from build123d import *

# Parameters (mm, degrees)
F1_DEPTH  = 6
F3_DEPTH  = 0.5
F5_DEPTH  = 0.5
F6_R      = 2.99999
F7_R      = 2.99999
F9_DEPTH  = 2
F10_DEPTH = 0.25
F11_R     = 0.75
F12_DEPTH = 2
F13_DEPTH = 0.25


# Not quite as in the source:
# - a fillet or chamfer is up to 0.001 mm smaller than in the source, because OpenCascade refuses the exact size


with BuildPart() as f1:
    # F0 (on Top) → F1 (new body)
    with BuildSketch(Plane.XY):
        with BuildLine():
            ThreePointArc((-21.257927263, 3.0925971456), (-19.5135237331, 1.2849088277), (-19.5663380414, -1.2266427602))
            ThreePointArc((-19.5663380414, -1.2266427602), (-17.0596555887, 1.5276447909), (-13.757927263, 3.2504758611))
            Line((-13.757927263, 3.2504758611), (-13.757927263, 16.4425971456))
            Line((-13.757927263, 16.4425971456), (-21.257927263, 12.0925971456))
            Line((-21.257927263, 12.0925971456), (-21.257927263, 3.0925971456))
        make_face()
        with BuildLine():
            ThreePointArc((-19.937029438, -1.8621137259), (-13.1593751133, -17.2347921219), (0.092072737, -6.9074028544))
            ThreePointArc((0.092072737, -6.9074028544), (-0.2305379955, -4.3059550041), (-1.178825088, -1.8621137259))
            ThreePointArc((-1.178825088, -1.8621137259), (-1.3821012217, -1.5548376637), (-1.5495164847, -1.2266427602))
            ThreePointArc((-1.5495164847, -1.2266427602), (-4.0561989374, 1.5276447909), (-7.357927263, 3.2504758611))
            Line((-7.357927263, 3.2504758611), (-7.357927263, 1.1925971456))
            Line((-7.357927263, 1.1925971456), (-7.357927263, 0.9928541258))
            Line((-7.357927263, 0.9928541258), (-10.557927263, 0.9928541258))
            Line((-10.557927263, 0.9928541258), (-13.757927263, 0.9928541258))
            Line((-13.757927263, 0.9928541258), (-13.757927263, 1.1925971456))
            Line((-13.757927263, 1.1925971456), (-13.757927263, 3.2504758611))
            ThreePointArc((-13.757927263, 3.2504758611), (-17.0596555887, 1.5276447909), (-19.5663380414, -1.2266427602))
            ThreePointArc((-19.5663380414, -1.2266427602), (-19.7337533043, -1.5548376637), (-19.937029438, -1.8621137259))
        make_face()
        with BuildLine():
            ThreePointArc((-7.407927263, -6.9074028544), (-12.7853136237, -9.1347892152), (-10.557927263, -3.7574028544))
            ThreePointArc((-10.557927263, -3.7574028544), (-8.3305409023, -4.6800164937), (-7.407927263, -6.9074028544))
        make_face(mode=Mode.SUBTRACT)
        with BuildLine():
            ThreePointArc((-7.357927263, 3.2504758611), (-4.0561989374, 1.5276447909), (-1.5495164847, -1.2266427602))
            ThreePointArc((-1.5495164847, -1.2266427602), (-1.6023307929, 1.2849088277), (0.142072737, 3.0925971456))
            Line((0.142072737, 3.0925971456), (0.142072737, 12.0925971456))
            Line((0.142072737, 12.0925971456), (-7.357927263, 16.4425971456))
            Line((-7.357927263, 16.4425971456), (-7.357927263, 3.2504758611))
        make_face()
    extrude(amount=F1_DEPTH)

    # F2 (on face) → F3 (join)
    with BuildSketch(Plane.YZ.offset(-13.757927263)):
        with BuildLine():
            ThreePointArc((11.9425971456, 0), (14.0639174891, 0.8786796564), (14.9425971456, 3))
            ThreePointArc((14.9425971456, 3), (14.0639174891, 5.1213203436), (11.9425971456, 6))
            ThreePointArc((11.9425971456, 6), (8.9425971456, 3), (11.9425971456, 0))
        make_face()
    extrude(amount=F3_DEPTH)

    # F4 (on face) → F5 (join)
    with BuildSketch(Plane(origin=(-7.357927263, 0, 0), x_dir=(0, -1, 0), z_dir=(-1, 0, 0))):
        with BuildLine():
            ThreePointArc((-11.9425971456, 0), (-9.821276802, 0.8786796564), (-8.9425971456, 3))
            ThreePointArc((-8.9425971456, 3), (-9.821276802, 5.1213203436), (-11.9425971456, 6))
            ThreePointArc((-11.9425971456, 6), (-14.9425971456, 3), (-11.9425971456, 0))
        make_face()
    extrude(amount=F5_DEPTH)

    # F6 (radius 3 in the source; OpenCascade refuses exactly that, so slightly less here)
    f6_edges = [f1.edges().sort_by_distance(p)[0] for p in [
        (-10.557927, 0.992854, 0),
        (-10.557927, 0.992854, 6),
    ]]
    fillet(f6_edges, radius=F6_R)

    # F7 (radius 3 in the source; OpenCascade refuses exactly that, so slightly less here)
    f7_edges = [f1.edges().sort_by_distance(p)[0] for p in [
        (-3.607927, 14.267597, 6),
        (-3.607927, 14.267597, 0),
        (-17.507927, 14.267597, 6),
        (-17.507927, 14.267597, 0),
    ]]
    fillet(f7_edges, radius=F7_R)

    # F8 (on face) → F9 (cut)
    with BuildSketch(Plane.XY.offset(6)):
        with BuildLine():
            ThreePointArc((-10.557927263, -13.8074028544), (-12.057927263, -15.3074028544), (-10.557927263, -16.8074028544))
            Line((-10.557927263, -16.8074028544), (-10.557927263, -16.0574028544))
            ThreePointArc((-10.557927263, -16.0574028544), (-11.307927263, -15.3074028544), (-10.557927263, -14.5574028544))
            Line((-10.557927263, -14.5574028544), (-10.557927263, -13.8074028544))
        make_face()
        with BuildLine():
            ThreePointArc((-7.557927263, -13.8074028544), (-8.4366069195, -11.6860825109), (-10.557927263, -10.8074028544))
            ThreePointArc((-10.557927263, -10.8074028544), (-9.057927263, -12.3074028544), (-10.557927263, -13.8074028544))
            Line((-10.557927263, -13.8074028544), (-10.557927263, -14.5574028544))
            ThreePointArc((-10.557927263, -14.5574028544), (-10.0275971771, -14.7770727685), (-9.807927263, -15.3074028544))
            ThreePointArc((-9.807927263, -15.3074028544), (-10.0275971771, -15.8377329403), (-10.557927263, -16.0574028544))
            Line((-10.557927263, -16.0574028544), (-10.557927263, -16.8074028544))
            ThreePointArc((-10.557927263, -16.8074028544), (-8.4366069195, -15.928723198), (-7.557927263, -13.8074028544))
        make_face()
        with BuildLine():
            Line((-10.557927263, -13.0574028544), (-10.557927263, -11.5574028544))
            ThreePointArc((-10.557927263, -11.5574028544), (-11.307927263, -12.3074028544), (-10.557927263, -13.0574028544))
        make_face()
        with BuildLine():
            ThreePointArc((-9.807927263, -12.3074028544), (-10.0275971771, -11.7770727685), (-10.557927263, -11.5574028544))
            Line((-10.557927263, -11.5574028544), (-10.557927263, -13.0574028544))
            ThreePointArc((-10.557927263, -13.0574028544), (-10.0275971771, -12.8377329403), (-9.807927263, -12.3074028544))
        make_face()
    extrude(amount=-F9_DEPTH, mode=Mode.SUBTRACT)

    # F8 (on face) → F10 (cut)
    with BuildSketch(Plane.XY.offset(6)):
        with BuildLine():
            Line((-10.557927263, -11.5574028544), (-10.557927263, -10.8074028544))
            ThreePointArc((-10.557927263, -10.8074028544), (-13.557927263, -13.8074028544), (-10.557927263, -16.8074028544))
            ThreePointArc((-10.557927263, -16.8074028544), (-12.057927263, -15.3074028544), (-10.557927263, -13.8074028544))
            Line((-10.557927263, -13.8074028544), (-10.557927263, -13.0574028544))
            ThreePointArc((-10.557927263, -13.0574028544), (-11.307927263, -12.3074028544), (-10.557927263, -11.5574028544))
        make_face()
        with BuildLine():
            ThreePointArc((-10.557927263, -13.8074028544), (-9.057927263, -12.3074028544), (-10.557927263, -10.8074028544))
            Line((-10.557927263, -10.8074028544), (-10.557927263, -11.5574028544))
            ThreePointArc((-10.557927263, -11.5574028544), (-10.0275971771, -11.7770727685), (-9.807927263, -12.3074028544))
            ThreePointArc((-9.807927263, -12.3074028544), (-10.0275971771, -12.8377329403), (-10.557927263, -13.0574028544))
            Line((-10.557927263, -13.0574028544), (-10.557927263, -13.8074028544))
        make_face()
        with BuildLine():
            Line((-10.557927263, -14.5574028544), (-10.557927263, -16.0574028544))
            ThreePointArc((-10.557927263, -16.0574028544), (-10.0275971771, -15.8377329403), (-9.807927263, -15.3074028544))
            ThreePointArc((-9.807927263, -15.3074028544), (-10.0275971771, -14.7770727685), (-10.557927263, -14.5574028544))
        make_face()
        with BuildLine():
            ThreePointArc((-10.557927263, -14.5574028544), (-11.307927263, -15.3074028544), (-10.557927263, -16.0574028544))
            Line((-10.557927263, -16.0574028544), (-10.557927263, -14.5574028544))
        make_face()
    extrude(amount=-F10_DEPTH, mode=Mode.SUBTRACT)

    # F11 (on face) → F12 (cut)
    with BuildSketch(Plane(origin=(0, 0, 0), x_dir=(1, 0, 0), z_dir=(0, 0, -1))):
        with BuildLine():
            ThreePointArc((-10.557927263, 13.8074028544), (-12.057927263, 15.3074028544), (-10.557927263, 16.8074028544))
            ThreePointArc((-10.557927263, 16.8074028544), (-13.557927263, 13.8074028544), (-10.557927263, 10.8074028544))
            ThreePointArc((-10.557927263, 10.8074028544), (-9.057927263, 12.3074028544), (-10.557927263, 13.8074028544))
        make_face()
        with Locations((-10.557927263, 12.3074028544)):
            Circle(F11_R, mode=Mode.SUBTRACT)
        with Locations((-10.557927263, 15.3074028544)):
            Circle(F11_R)
    extrude(amount=-F12_DEPTH, mode=Mode.SUBTRACT)

    # F11 (on face) → F13 (cut)
    with BuildSketch(Plane(origin=(0, 0, 0), x_dir=(1, 0, 0), z_dir=(0, 0, -1))):
        with BuildLine():
            ThreePointArc((-10.557927263, 10.8074028544), (-8.4366069195, 11.6860825109), (-7.557927263, 13.8074028544))
            ThreePointArc((-7.557927263, 13.8074028544), (-8.4366069195, 15.928723198), (-10.557927263, 16.8074028544))
            ThreePointArc((-10.557927263, 16.8074028544), (-12.057927263, 15.3074028544), (-10.557927263, 13.8074028544))
            ThreePointArc((-10.557927263, 13.8074028544), (-9.057927263, 12.3074028544), (-10.557927263, 10.8074028544))
        make_face()
        with Locations((-10.557927263, 15.3074028544)):
            Circle(F11_R, mode=Mode.SUBTRACT)
        with Locations((-10.557927263, 12.3074028544)):
            Circle(F11_R)
    extrude(amount=-F13_DEPTH, mode=Mode.SUBTRACT)


solid = f1.part
Could you check a few things on this model? Use its own coordinates, in mm. A direction names the side the tool comes from. Round coordinates to 2 decimals unless told otherwise and drop trailing zeros. Order: outer loops, then holes, each group sorted by start corner. A loop starts at its lowest first (then second) coordinate and runs counter-clockwise, first axis right, second up. Notation, with made-up numbers: M 3,-27 L 23,-27 A34 ccw 23,3 Z; hole C 39,16 d5. An arc over 180 degrees is marked long. One line per item, written item: value.
(1) If we mould it in two halves opening along X, with no side actions, what happens to faces 4 (the cylindrical face through (-17.871, 13.014, 0.855)), 5 (the flat face through (-13.758, 5, 3)), 6 (the flat face through (0.142, 8, 3))? For each: released by +X, released by -X, zero draft, split by the parting line, or undercut.
Ans:
face 4: released by -X
face 5: undercut
face 6: released by +X
(2) Imagine slicing it at C-C (z = 3.5). Write out the boundary of the cut face in (x, y), and give its area (3 significant figures).
Ans:
outline: M -21.26,3.09 A3.27 cw -19.94,-1.86 A10.65 ccw long -1.18,-1.86 A3.27 cw 0.14,3.09 L 0.14,12.04 L -7.36,16.39 L -7.36,14.9 L -7.86,14.9 L -7.86,8.98 L -7.36,8.98 L -7.36,0.95 L -13.76,0.95 L -13.76,8.98 L -13.26,8.98 L -13.26,14.9 L -13.76,14.9 L -13.76,16.39 L -21.26,12.04 Z; hole C -10.56,-6.91 d6.3
area: 500 mm^2
(3) Imagine slicing it at D-D (y = 4.5). Write out the boundary of the cut face in (x, z).
Ans:
outline: M -21.26,0 L -13.76,0 L -13.76,6 L -21.26,6 Z; M -7.36,0 L 0.14,0 L 0.14,6 L -7.36,6 Z
(4) Which directions (+Z, -Z, +X, -X, +Y, -Y) give clear straight access to the entire face, cutting with the end or side of a thin tool? Please do faces 1 (the flat face through (-11, -12, 0.25)), 2 (the flat face through (-11.3, -13.1, 5.75)), 3 (the flat face through (-7.358, 15.2, 3)).
Ans:
face 1: -Z
face 2: +Z
face 3: +Z, +Y
(5) Imagine slicing it at A-A (y = -6.5). Write out the boundary of the cut face in (x, z), and give its area (3 significant figures).
Ans:
outline: M -21.2,0 L -13.68,0 L -13.68,6 L -21.2,6 Z; M -7.43,0 L 0.08,0 L 0.08,6 L -7.43,6 Z
area: 90.2 mm^2
(6) I'm going to push flat-ended pins straight in: P1, Ø1.5, axis at x = -6.5, z = 5, coming from the +Y side; P2, Ø2, axis at x = -4.5, z = 5, coming from the -Y side; P3, Ø0.8, axis at x = -10.5, y = -12.5, coming from the +Z side. Where does each tip first touch, or does it pass through?
Ans:
P1: stops at y = 15.81
P2: stops at y = -16.28
P3: stops at z = 4
(7) I need wall thicknesses on line 1 along X through (y, z) = (-15, 0.75); line 2 along Y through (x, z) = (-7.75, 1) (3 decimals); line 3 along X through (y, z) = (10.5, 5.5). Which ranges of each line are inside material? Lowest first, please. Write a range as from..to.
Ans:
line 1: x = -17.48..-13.31, -12.03..-11.24, -9.87..-3.63
line 2: y = -17.181..-8.335, -5.48..0.229, 9.707..14.179
line 3: x = -21.26..-13.26, -7.86..0.14
